For this review, use the dimensioned drawing (mm, ordinates from the lowest corner) and the shaded views. A direction names the side the tool comes from. Give positions to 0.01 mm unless a question says otherwise; leave off trailing zeros. Write each loop counter-clockwise with the first axis right and the second up, starting at its lowest first coordinate (ties: lowest second). Pieces come first, ordered by that corner, then holes. Notation, with made-up numbers: (35.25, 30.5) -> (78.25, 30.5) arc R16 ccw to (78.25, 40.5) -> close; hole circle Ø5 at (1.5, -10). An arc over 180 degrees is marked (long way). Write each question's results on one line, items separated by ' | '. Start each with the question number.
(1) Clearance check with a flat-ended pin moving along its axis: pin 1 (6 mm diameter, centred on x = 36.5, z = 35, fed in from -Y). State where the tip first meets the part, or that it passes through.
(2) Take a section at C-C (x = 174.5). State the section outline as (y, z) points.
(3) Take a section at A-A (y = 201). State the section outline as (x, z) points.
(4) Take a section at B-B (z = 27). State the section outline as (x, y) points.
(5) To check wall thickness, follow probe 1 along Y at (x, z) = (149, 32); probe 2 along X at (y, z) = (210, 17). State the ranges of each line that lie inside material, in increasing order.
(6) For the marked faces 5 and 6, list the 3-axis set-ups (+Z, -Z, +X, -X, +Y, -Y) from which the entire face can be reached by the end or side of a thin tool; tool diameter is ignored.
(7) Mouldability with a two-part tool opening along X and no side actions: class the marked faces 1, 2, 3 and 4 as released by +X, released by -X, zero draft, split by the parting line, or undercut.
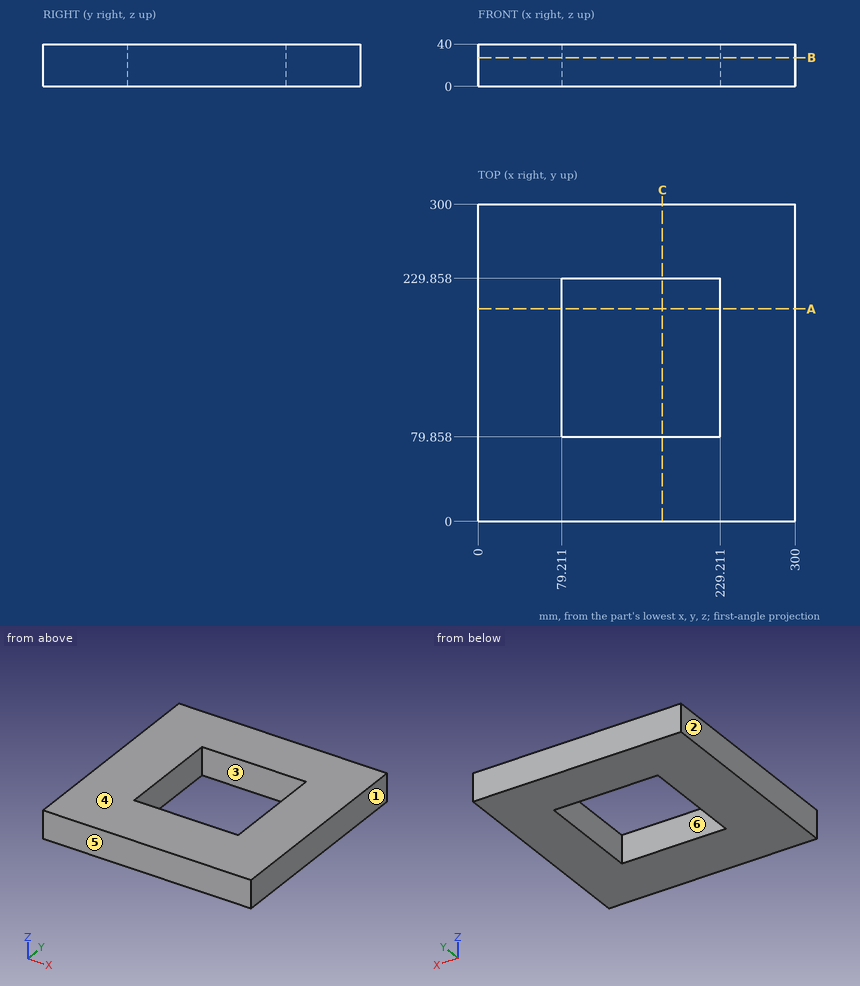
Report:
1) pin 1: y = 0
2) outline: (0, 0) -> (79.86, 0) -> (79.86, 40) -> (0, 40) -> close; (229.86, 0) -> (300, 0) -> (300, 40) -> (229.86, 40) -> close
3) outline: (0, 0) -> (79.21, 0) -> (79.21, 40) -> (0, 40) -> close; (229.21, 0) -> (300, 0) -> (300, 40) -> (229.21, 40) -> close
4) outline: (0, 0) -> (300, 0) -> (300, 300) -> (0, 300) -> close; hole (79.21, 79.86) -> (229.21, 79.86) -> (229.21, 229.86) -> (79.21, 229.86) -> close
5) probe 1: 0 to 79.86, 229.86 to 300 | probe 2: 0 to 79.21, 229.21 to 300
6) face 5: +Z, -Z, +X, -X, -Y | face 6: +Z, -Z
7) face 1: released by +X | face 2: released by -X | face 3: undercut | face 4: zero draft
